from build123d import *

# Parameters (mm, degrees)
F0_R     = 12.7
F1_DEPTH = 25.4
F2_DEPTH = 50.8


# Not quite as in the source:
# - a feature names something its author has since deleted; it is built from what else it names


with BuildPart() as f1:
    # F0 (on Front) → F1 (new body)
    with BuildSketch(Plane.XZ):
        with BuildLine():
            ThreePointArc((4.7257233878, 37.8057871028), (28.5627384986, 25.2146776593), (38.1, 0))
            ThreePointArc((38.1, 0), (28.5627384986, -25.2146776593), (4.7257233878, -37.8057871028))
            Line((4.7257233878, -37.8057871028), (105.541155662, -25.2038580685))
            ThreePointArc((105.541155662, -25.2038580685), (76.9906734034, 0), (105.541155662, 25.2038580685))
            Line((105.541155662, 25.2038580685), (4.7257233878, 37.8057871028))
        make_face()
        with BuildLine():
            ThreePointArc((127.7906734034, 0), (121.4324990691, 16.8097851062), (105.541155662, 25.2038580685))
            ThreePointArc((105.541155662, 25.2038580685), (76.9906734034, 0), (105.541155662, -25.2038580685))
            ThreePointArc((105.541155662, -25.2038580685), (121.4324990691, -16.8097851062), (127.7906734034, 0))
        make_face()
        with Locations((102.3906734034, 0)):
            Circle(F0_R, mode=Mode.SUBTRACT)
        with BuildLine():
            ThreePointArc((4.7257233878, -37.8057871028), (28.5627384986, -25.2146776593), (38.1, 0))
            ThreePointArc((38.1, 0), (28.5627384986, 25.2146776593), (4.7257233878, 37.8057871028))
            ThreePointArc((4.7257233878, 37.8057871028), (-38.1, 0), (4.7257233878, -37.8057871028))
        make_face()
        with BuildLine():
            ThreePointArc((-17.3665807845, 7.8297108412), (0, 19.05), (17.3665807845, 7.8297108412))
            Line((17.3665807845, 7.8297108412), (27.8837817341, 7.8297108412))
            Line((27.8837817341, 7.8297108412), (27.8837817341, -7.8297108412))
            Line((27.8837817341, -7.8297108412), (17.3665807845, -7.8297108412))
            ThreePointArc((17.3665807845, -7.8297108412), (0, -19.05), (-17.3665807845, -7.8297108412))
            Line((-17.3665807845, -7.8297108412), (-22.9162182659, -7.8297108412))
            Line((-22.9162182659, -7.8297108412), (-22.9162182659, 0))
            Line((-22.9162182659, 0), (-22.9162182659, 7.8297108412))
            Line((-22.9162182659, 7.8297108412), (-17.3665807845, 7.8297108412))
        make_face(mode=Mode.SUBTRACT)
        with BuildLine():
            ThreePointArc((-17.3665807845, -7.8297108412), (-19.05, 0), (-17.3665807845, 7.8297108412))
            Line((-17.3665807845, 7.8297108412), (-22.9162182659, 7.8297108412))
            Line((-22.9162182659, 7.8297108412), (-22.9162182659, 0))
            Line((-22.9162182659, 0), (-22.9162182659, -7.8297108412))
            Line((-22.9162182659, -7.8297108412), (-17.3665807845, -7.8297108412))
        make_face()
    extrude(amount=F1_DEPTH)

    # F0 (on Front) → F2 (join)
    with BuildSketch(Plane.XZ):
        with BuildLine():
            ThreePointArc((4.7257233878, -37.8057871028), (28.5627384986, -25.2146776593), (38.1, 0))
            ThreePointArc((38.1, 0), (28.5627384986, 25.2146776593), (4.7257233878, 37.8057871028))
            ThreePointArc((4.7257233878, 37.8057871028), (-38.1, 0), (4.7257233878, -37.8057871028))
        make_face()
        with BuildLine():
            ThreePointArc((-17.3665807845, 7.8297108412), (0, 19.05), (17.3665807845, 7.8297108412))
            Line((17.3665807845, 7.8297108412), (27.8837817341, 7.8297108412))
            Line((27.8837817341, 7.8297108412), (27.8837817341, -7.8297108412))
            Line((27.8837817341, -7.8297108412), (17.3665807845, -7.8297108412))
            ThreePointArc((17.3665807845, -7.8297108412), (0, -19.05), (-17.3665807845, -7.8297108412))
            Line((-17.3665807845, -7.8297108412), (-22.9162182659, -7.8297108412))
            Line((-22.9162182659, -7.8297108412), (-22.9162182659, 0))
            Line((-22.9162182659, 0), (-22.9162182659, 7.8297108412))
            Line((-22.9162182659, 7.8297108412), (-17.3665807845, 7.8297108412))
        make_face(mode=Mode.SUBTRACT)
        with BuildLine():
            ThreePointArc((-17.3665807845, -7.8297108412), (-19.05, 0), (-17.3665807845, 7.8297108412))
            Line((-17.3665807845, 7.8297108412), (-22.9162182659, 7.8297108412))
            Line((-22.9162182659, 7.8297108412), (-22.9162182659, 0))
            Line((-22.9162182659, 0), (-22.9162182659, -7.8297108412))
            Line((-22.9162182659, -7.8297108412), (-17.3665807845, -7.8297108412))
        make_face()
    extrude(amount=F2_DEPTH)


solid = f1.part
Could you check a few things on this model? Use its own coordinates, in mm. A direction names the side the tool comes from. Round coordinates to 2 decimals unless told otherwise and drop trailing zeros. Order: outer loops, then holes, each group sorted by start corner. A loop starts at its lowest first (then second) coordinate and runs counter-clockwise, first axis right, second up. Notation, with made-up numbers: M 64,-28 L 69,-28 A16 ccw 69,-12 Z; hole C 55,32 d3. An arc over 180 degrees is marked long. One line per item, written item: value.
(1) If we mould it in two halves opening along Z, with no side actions, what happens to faces 3 (the flat face through (23, -25, -7.83)), 4 (the cylindrical face through (-19.036, -25.044, -0.725)), 5 (the cylindrical face through (-37.93, -30.69, 3.58)), 6 (the flat face through (54.428, -12.522, -31.593))? For each: released by +Z, released by -Z, zero draft, split by the parting line, or undercut.
Ans:
face 3: undercut
face 4: undercut
face 5: split by the parting line
face 6: released by -Z
(2) Imagine slicing it at A-A (z = 0). Write out the boundary of the cut face in (x, y), and give its area (3 significant figures).
Ans:
outline: M -38.1,-50.8 L -19.05,-50.8 L -19.05,0 L -38.1,0 Z; M 27.88,-50.8 L 38.1,-50.8 L 38.1,-25.4 L 89.69,-25.4 L 89.69,0 L 27.88,0 Z; M 115.09,-25.4 L 127.79,-25.4 L 127.79,0 L 115.09,0 Z
area: 3,120 mm^2
(3) Which directions (+Z, -Z, +X, -X, +Y, -Y) give clear straight access to the entire face, cutting with the end or side of a thin tool? Please do faces 1 (the flat face through (55.839, -12.522, 31.417)), 2 (the flat face through (23, -25, 7.83)).
Ans:
face 1: +Z, +X, +Y, -Y
face 2: +Y, -Y
(4) I need wall thicknesses on line 1 along Z through (x, y) = (0, -16); line 2 along X through (y, z) = (-27.5, 0); line 3 along X through (y, z) = (-6, 8). Which ranges of each line are inside material? Lowest first, please. Write a range as from..to.
Ans:
line 1: z = -38.1..-19.05, 19.05..38.1
line 2: x = -38.1..-19.05, 27.88..38.1
line 3: x = -37.25..-17.29, 17.29..92.53, 112.25..126.5
(5) Imagine slicing it at D-D (x = 30). Write out the boundary of the cut face in (y, z).
Ans:
outline: M -50.8,-23.49 L -25.4,-23.49 L -25.4,-34.65 L 0,-34.65 L 0,34.65 L -25.4,34.65 L -25.4,23.49 L -50.8,23.49 Z
(6) Imagine slicing it at C-C (x = 0). Write out the boundary of the cut face in (y, z), and give its area (3 significant figures).
Ans:
outline: M -50.8,-38.1 L 0,-38.1 L 0,-19.05 L -50.8,-19.05 Z; M -50.8,19.05 L 0,19.05 L 0,38.1 L -50.8,38.1 Z
area: 1,940 mm^2
(7) Imagine slicing it at B-B (y = -20). Write out the boundary of the cut face in (x, z), and give its area (3 significant figures).
Ans:
outline: M 4.73,-37.81 L 105.54,-25.2 A25.4 ccw 105.54,25.2 L 4.73,37.81 A38.1 ccw long Z; hole M 17.37,-7.83 L 27.88,-7.83 L 27.88,7.83 L 17.37,7.83 A19.05 ccw long Z; hole C 102.39,0 d25.4
area: 8,050 mm^2
(8) I'm going to push flat-ended pins straight in: P1, Ø8, axis at y = -44, z = -6, coming from the +X side; P2, Ø4, axis at y = -37, z = 21.5, coming from the +X side; P3, Ø4, axis at x = 61.5, y = -12, coming from the +Z side. Where does each tip first touch, or does it pass through?
Ans:
P1: stops at x = 38.05
P2: stops at x = 32.73
P3: stops at z = 30.96
